Geometry check sheet. Reference: the model listing, model coordinates, mm. A direction names the side the tool comes from. Round coordinates to 2 decimals unless told otherwise and drop trailing zeros. Loops run counter-clockwise (first coordinate to the right, second up) from the corner with the lowest first, then second, coordinate; pieces in that order, holes last. Notation, with made-up numbers: (70.25, 78) - (120.25, 78) arc R9 cw to (120.25, 94) - close; hole circle Ø11 at (67, -32.5). An arc over 180 degrees is marked (long way). Write item = value, one per line.
```python
from build123d import *

# Parameters (mm, degrees)
F0_W        = 129.5146
F0_H        = 11.303
F1_DEPTH    = 9.271
F2_W        = 206.3660303733
F2_H        = 3.175
F3_DEPTH    = 7.5438
F4_W        = 3.7084
F4_H        = 3.175
F5_DEPTH    = 25.4
F6_W        = 16.3322
F6_H        = 3.175
F7_DEPTH    = 25.4
F8_T1_DEPTH = 29.464
F8_T3_DEPTH = 29.464
F9_R        = 1.524
F10_DEPTH   = 25.4
F12_DEPTH   = 25.4
F13_W       = 11.2141259015
F13_H       = 1.2269735361
F14_DEPTH   = 4.1656
F15_DEPTH   = 0.254
F16_DEPTH   = 3.175
F16_FACE_W  = 4.4019735361
F16_FACE_H  = 4.1656
F17_ANGLE   = 90


# Not quite as in the source:
# - a fillet or chamfer that OpenCascade refuses, or shapes differently, is made with other operations: its cross-section is extruded or revolved along the edge and cut away or added


with BuildPart() as f1:
    # F0 (on Top) → F1 (new body)
    with BuildSketch(Plane.XY):
        Rectangle(F0_W, F0_H)
    extrude(amount=F1_DEPTH)

    # F2 (on face) → F3 (cut)
    with BuildSketch(Plane.XY.offset(9.271)):
        Rectangle(F2_W, F2_H)
    extrude(amount=-F3_DEPTH, mode=Mode.SUBTRACT)

    # F4 (on face) → F5 (cut)
    with BuildSketch(Plane.XY.offset(1.7272)):
        with Locations((62.9031, 0)):
            Rectangle(F4_W, F4_H)
    extrude(amount=-F5_DEPTH, mode=Mode.SUBTRACT)

    # F6 (on face) → F7 (cut)
    with BuildSketch(Plane.XY.offset(1.7272)):
        with Locations((-56.5912, 0)):
            Rectangle(F6_W, F6_H)
    extrude(amount=-F7_DEPTH, mode=Mode.SUBTRACT)

    # F8: fillet of radius 5.08 on 4 edges, made by hand

    # F8_s2 → F8_t1 (cut)
    with BuildSketch(Plane.XZ.offset(-11.1125)):
        with BuildLine():
            ThreePointArc((-64.7573, 4.191), (-63.2694024484, 7.7831024484), (-59.6773, 9.271))
            Line((-59.6773, 9.271), (-64.7573, 9.271))
            Line((-64.7573, 9.271), (-64.7573, 4.191))
        make_face()
        with BuildLine():
            ThreePointArc((-64.7573, 5.08), (-63.2694024484, 1.4878975516), (-59.6773, 0))
            Line((-59.6773, 0), (-64.7573, 0))
            Line((-64.7573, 0), (-64.7573, 5.08))
        make_face()
    extrude(amount=F8_T1_DEPTH, mode=Mode.SUBTRACT)

    # F8_s4 → F8_t3 (cut)
    with BuildSketch(Plane.XZ.offset(-18.3515)):
        with BuildLine():
            ThreePointArc((-59.6773, 9.271), (-63.2694024484, 7.7831024484), (-64.7573, 4.191))
            Line((-64.7573, 4.191), (-64.7573, 9.271))
            Line((-64.7573, 9.271), (-59.6773, 9.271))
        make_face()
        with BuildLine():
            ThreePointArc((-64.7573, 5.08), (-63.2694024484, 1.4878975516), (-59.6773, 0))
            Line((-59.6773, 0), (-64.7573, 0))
            Line((-64.7573, 0), (-64.7573, 5.08))
        make_face()
    extrude(amount=F8_T3_DEPTH, mode=Mode.SUBTRACT)

    # F9 (on face) → F10 (cut)
    with BuildSketch(Plane.XZ.offset(5.6515)):
        with Locations((-61.0294157593, 4.6167229302)):
            Circle(F9_R)
    extrude(amount=-F10_DEPTH, mode=Mode.SUBTRACT)

    # F11 (on face) → F12 (cut)
    with BuildSketch(Plane.XZ.offset(5.6515)):
        with BuildLine():
            Line((61.4553, 4.6355), (63.9953, 4.6355))
            ThreePointArc((63.9953, 4.6355), (62.7253, 5.9055), (61.4553, 4.6355))
        make_face()
        with BuildLine():
            ThreePointArc((61.4553, 4.6355), (62.7253, 3.3655), (63.9953, 4.6355))
            Line((63.9953, 4.6355), (61.4553, 4.6355))
        make_face()
    extrude(amount=-F12_DEPTH, mode=Mode.SUBTRACT)


with BuildPart() as f14:
    # F13 (on Top) → F14 (new body)
    with BuildSketch(Plane.XY):
        with Locations((67.7984524518, -0.613486768)):
            Rectangle(F13_W, F13_H)
    extrude(amount=F14_DEPTH)


with BuildPart() as f15:
    # F15 (new): a face of the model
    f15_faces = [f14.part.faces().sort_by_distance(p)[0] for p in [
        (73.4055154026, -0.613486768, 2.0828),
    ]]
    extrude(f15_faces, amount=F15_DEPTH)


with BuildPart() as f14_1:
    add(f14.part)

    # F16 (add): a face of the model
    f16_faces = [f15.part.faces().sort_by_distance(p)[0] for p in [
        (73.5325154026, -1.2269735361, 2.0828),
    ]]

    add(f15.part)  # F16 merges F15
    extrude(f16_faces, amount=F16_DEPTH)


with BuildPart() as f17:
    # F16_face (on face) → F17 (revolve)
    with BuildSketch(Plane(origin=(73.6595154026, -2.200986768, 2.0828), x_dir=(0, 1, 0), z_dir=(1, 0, 0))):
        Rectangle(F16_FACE_W, F16_FACE_H)
    revolve(axis=Axis((73.6595154026, -2.200986768, 0), (0, -1, 0)), revolution_arc=F17_ANGLE)


with BuildPart() as f18_1:
    # F18: instance of F14
    add(f14_1.part.mirror(Plane.XZ))


with BuildPart() as f18_2:
    # F18: instance of F17
    add(f17.part.mirror(Plane.XZ))


solid = f1.part
```
(1) Mould release check, pull along X, two halves, no side actions. Record for faces 3 (the cylindrical face through (-63.15, -3.59, 7.9)), 4 (the flat face through (2, 4, 9.271)), 5 (the cylindrical face through (-62.552, -3.648, 4.684)), 6 (the flat face through (64.757, 4, 5)): pulls with the +X half, pulls with the -X half, needs draft (parallel to the pull), parting line crosses it, or undercut.
Answers follow:
face_3 = pulls with the -X half
face_4 = needs draft
face_5 = undercut
face_6 = pulls with the +X half
(2) Set-up check for faces 1 (the flat face through (2, -4, 9.271)), 2 (the flat face through (6, 0, 1.727)): record each of +Z, -Z, +X, -X, +Y, -Y from which the full face is reachable in a straight line by a thin tool's end or side.
Answers follow:
face_1 = +Z, +X, -X, +Y, -Y
face_2 = +Z, +X, -X
(3) Section check A-A (z = 7.75). Enter the section's corners in (x, y).
Answers follow:
outline = (-63.3, -5.65) - (64.76, -5.65) - (64.76, -1.59) - (-63.3, -1.59) - close; (-63.3, 1.59) - (64.76, 1.59) - (64.76, 5.65) - (-63.3, 5.65) - close
(4) Gauge pin test, flat ends, axial feed: pin 1 (1 mm diameter, centred on x = 12, y = -0.5, fed in from +Z); pin 2 (1.4 mm diameter, centred on y = 0, z = 1, fed in from -X); pin 3 (1.8 mm diameter, centred on x = -61.03, z = 4.62, fed in from -Y); pin 4 (0.5 mm diameter, centred on y = -0.5, z = 0.5, fed in from +X). Record the tip position at first contact, or that the pin passes through.
Answers follow:
pin_1 = 1.73
pin_2 = -48.43
pin_3 = through
pin_4 = 61.05
(5) Section check C-C (y = -4). Enter the section's corners in (x, z).
Answers follow:
outline = (-64.74, 4.64) arc R5.08 ccw to (-59.68, 0) - (64.76, 0) - (64.76, 9.27) - (-59.68, 9.27) arc R5.08 ccw to start; hole circle Ø3.05 at (-61.03, 4.62); hole circle Ø2.54 at (62.73, 4.64)
(6) Section check B-B (x = -41). Enter the section's corners in (y, z).
Answers follow:
outline = (-5.65, 0) - (5.65, 0) - (5.65, 9.27) - (1.59, 9.27) - (1.59, 1.73) - (-1.59, 1.73) - (-1.59, 9.27) - (-5.65, 9.27) - close
(7) Scan lines: L1, parallel to Y at x = 57.5, z = 6.25; L2, parallel to X at y = 5, z = 5.25; L3, parallel to Z at x = -15.5, y = -0.5. Record each from-to range of solid material in increasing order. Write a range as [from, to].
Answers follow:
L1 = [-5.65, -1.59], [1.59, 5.65]
L2 = [-64.65, -62.42], [-59.64, 61.61], [63.84, 64.76]
L3 = [0, 1.73]
